Check sheet for the modelled part. Datum: model origin and axes. Units: mm. Face numbers are marked on the shaded views. A direction names the side the tool comes from. Give positions to 0.01 mm unless a question says otherwise; leave off trailing zeros. Order: outer loops, then holes, each group sorted by start corner. A loop starts at its lowest first (then second) coordinate and runs counter-clockwise, first axis right, second up. Notation, with made-up numbers: (-31, 79) -> (-3, 79) arc R14 ccw to (-3, 88) -> close; hole circle Ø4 at (-0.75, 50). An arc over 180 degrees is marked (long way). One line per question, with ' | ' between items. Start each with the question number.
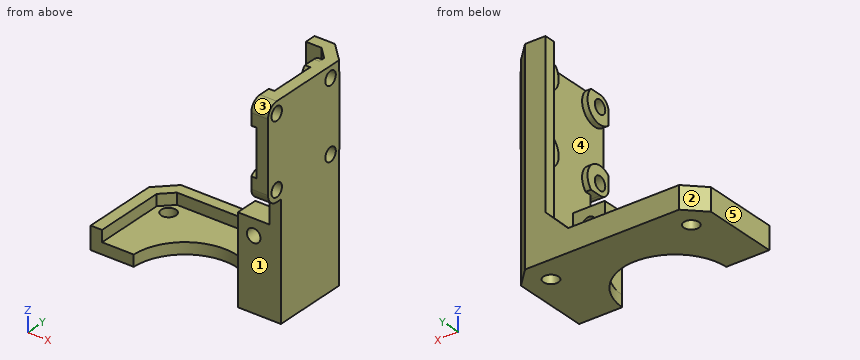
from build123d import *

# Parameters (mm, degrees)
BOSS_EXTRUDE1_DEPTH     = 2.5
SKETCH2_R               = 11.5
CUT_EXTRUDE1_DEPTH      = 3
SKETCH3_R               = 1.65
CUT_EXTRUDE2_DEPTH      = 3
EXTRUDE_THIN1_DEPTH     = 43.3
BOSS_EXTRUDE2_DEPTH     = 2.5
CUT_EXTRUDE3_DEPTH      = 57.003950753
CUT_EXTRUDE3_DEPTH_BACK = 57.003950753
SKETCH7_W               = 33.5
SKETCH7_H               = 40.8
CHAMFER1_SIZE           = 5
BOSS_EXTRUDE3_DEPTH     = 1.2
SKETCH10_R              = 1.5
CUT_EXTRUDE4_DEPTH      = 10
SKETCH12_W              = 9.502717712
SKETCH12_H              = 19.3
BOSS_EXTRUDE4_DEPTH     = 5
SKETCH13_R              = 1.5
CUT_EXTRUDE5_DEPTH      = 53.789227121


with BuildPart() as part:
    # Sketch1 → Boss-Extrude1 (new body)
    with BuildSketch(Plane.XY):
        Polygon((-21, 0.25), (21, 0.25), (21, 17), (17, 21), (-17, 21), (-21, 17), align=None)
    extrude(amount=BOSS_EXTRUDE1_DEPTH)

    # Sketch2 → Cut-Extrude1 (cut)
    with BuildSketch(Plane.XY.offset(2.5)):
        Circle(SKETCH2_R)
    extrude(amount=-CUT_EXTRUDE1_DEPTH, mode=Mode.SUBTRACT)

    # Sketch3 → Cut-Extrude2 (cut)
    with BuildSketch(Plane(origin=(0, 0, 0), x_dir=(-1, 0, 0), z_dir=(0, 0, -1))):
        with Locations((15.5, 15.5)):
            Circle(SKETCH3_R)
        with Locations((-15.5, 15.5)):
            Circle(SKETCH3_R)
    extrude(amount=-CUT_EXTRUDE2_DEPTH, mode=Mode.SUBTRACT)

    # Sketch4 → Extrude-Thin1 (add)
    with BuildSketch(Plane.XY.offset(2.5)):
        Polygon((21, 0.25), (21, 17), (17, 21), (-17, 21), (-21, 17), (-21, 0.25), (-18.5, 0.25), (-18.5, 15.964466094), (-15.964466094, 18.5), (15.964466094, 18.5), (18.5, 15.964466094), (18.5, 0.25), align=None)
    extrude(amount=EXTRUDE_THIN1_DEPTH)

    # Sketch6 → Boss-Extrude2 (add)
    with BuildSketch(Plane(origin=(21, 0, 0), x_dir=(0, 0, -1), z_dir=(1, 0, 0))):
        with BuildLine():
            Line((-45.8, 14.55), (-45.8, -0.95))
            ThreePointArc((-45.8, -0.95), (-45.067766953, -2.717766953), (-43.3, -3.45))
            Line((-43.3, -3.45), (-27.8, -3.45))
            ThreePointArc((-27.8, -3.45), (-26.032233047, -2.717766953), (-25.3, -0.95))
            Line((-25.3, -0.95), (-25.3, 14.55))
            ThreePointArc((-25.3, 14.55), (-26.032233047, 16.317766953), (-27.8, 17.05))
            Line((-27.8, 17.05), (-43.3, 17.05))
            ThreePointArc((-43.3, 17.05), (-45.067766953, 16.317766953), (-45.8, 14.55))
        make_face()
    extrude(amount=-BOSS_EXTRUDE2_DEPTH)

    # Sketch7 → Cut-Extrude3 (cut, two sides: drawn at the far end of the back side and taken through both)
    with BuildSketch(Plane(origin=(0, 21, 0), x_dir=(1, 0, 0), z_dir=(0, 1, 0)).offset(-CUT_EXTRUDE3_DEPTH_BACK)):
        with Locations((-4.25, -25.4)):
            Rectangle(SKETCH7_W, SKETCH7_H)
    extrude(amount=CUT_EXTRUDE3_DEPTH + CUT_EXTRUDE3_DEPTH_BACK, mode=Mode.SUBTRACT)

    # Chamfer1
    chamfer1_edges = [part.edges().sort_by_distance(p)[0] for p in [
        (12.5, 19.75, 5),
    ]]
    chamfer(chamfer1_edges, length=CHAMFER1_SIZE)

    # Sketch8 → Boss-Extrude3 (add)
    with BuildSketch(Plane.ZY.offset(-18.5)):
        with BuildLine():
            Line((27.8, -3.45), (30.390366769, -3.45))
            ThreePointArc((30.390366769, -3.45), (30.345584412, 1.595584412), (25.3, 1.640366769))
            Line((25.3, 1.640366769), (25.3, -0.95))
            ThreePointArc((25.3, -0.95), (26.032233047, -2.717766953), (27.8, -3.45))
        make_face()
        with BuildLine():
            Line((45.8, -0.95), (45.8, 1.640366769))
            ThreePointArc((45.8, 1.640366769), (40.754415588, 1.595584412), (40.709633231, -3.45))
            Line((40.709633231, -3.45), (43.3, -3.45))
            ThreePointArc((43.3, -3.45), (45.067766953, -2.717766953), (45.8, -0.95))
        make_face()
        with BuildLine():
            Line((43.3, 17.05), (40.709633231, 17.05))
            ThreePointArc((40.709633231, 17.05), (40.754415588, 12.004415588), (45.8, 11.959633231))
            Line((45.8, 11.959633231), (45.8, 14.55))
            ThreePointArc((45.8, 14.55), (45.067766953, 16.317766953), (43.3, 17.05))
        make_face()
        with BuildLine():
            Line((25.3, 14.55), (25.3, 11.959633231))
            ThreePointArc((25.3, 11.959633231), (30.345584412, 12.004415588), (30.390366769, 17.05))
            Line((30.390366769, 17.05), (27.8, 17.05))
            ThreePointArc((27.8, 17.05), (26.032233047, 16.317766953), (25.3, 14.55))
        make_face()
    extrude(amount=BOSS_EXTRUDE3_DEPTH)

    # Sketch10 → Cut-Extrude4 (cut)
    with BuildSketch(Plane.ZY.offset(-17.3)):
        with Locations((43.3, 14.55)):
            Circle(SKETCH10_R)
        with Locations((27.8, 14.55)):
            Circle(SKETCH10_R)
        with Locations((27.8, -0.95)):
            Circle(SKETCH10_R)
        with Locations((43.3, -0.95)):
            Circle(SKETCH10_R)
    extrude(amount=-CUT_EXTRUDE4_DEPTH, mode=Mode.SUBTRACT)

    # Sketch12 → Boss-Extrude4 (add)
    with BuildSketch(Plane.XZ.offset(-0.25)):
        with Locations((16.248641144, 9.65)):
            Rectangle(SKETCH12_W, SKETCH12_H)
    extrude(amount=-BOSS_EXTRUDE4_DEPTH)

    # Sketch13 → Cut-Extrude5 (cut, through all)
    with BuildSketch(Plane(origin=(0, 5.25, 0), x_dir=(1, 0, 0), z_dir=(0, 1, 0))):
        with Locations(Location((14.998641144, -15.8, 0), (0, 0, 270))):
            Circle(SKETCH13_R)
    extrude(amount=-CUT_EXTRUDE5_DEPTH, mode=Mode.SUBTRACT)


solid = part.part
1. Tool access check on the marked faces 1 and 2. Record the directions out of +Z, -Z, +X, -X, +Y, -Y that give a thin tool (end or side, any length) a straight path to the whole face; none if there is none.
2. Cross-section at C-C on x = 0. Record the boundary of the cut face in (y, z).
3. Cross-section at B-B on y = 4.5. Record the boundary of the cut face in (x, z), and give its area (3 significant figures).
4. Go/stop test with flat-tipped pins: pin 1 (6 mm diameter, centred on x = -2, y = 12.5, fed in from +Z); pin 2 (3 mm diameter, centred on y = 2.5, z = 30, fed in from -X); pin 3 (5 mm diameter, centred on x = 15, y = 7.5, fed in from +Z); pin 4 (8 mm diameter, centred on x = -15, y = 8, fed in from -Z). Record where each tip stops, or that it passes through.
5. Cross-section at D-D on z = 32. Record the boundary of the cut face in (x, y).
6. Cross-section at A-A on z = 15.8. Record the boundary of the cut face in (x, y), and give its area (3 significant figures).
7. Mould release check, pull along Z, two halves, no side actions. Record for the marked faces 3, 4 and 5: +Z half, -Z half, draft (parallel to the pull), parting line (faces both ways), or undercut.
8. Scan lines: probe 1 along X at (y, z) = (1, 3); probe 2 along X at (y, z) = (11.25, 4.5); probe 3 along Y at (x, z) = (15.5, 1.15). Record each from-to range of solid material in increasing order.
Response values:
1) face 1: -Z, +X, -X, -Y | face 2: +Z, -Z, -X, +Y
2) outline: (11.5, 0) -> (21, 0) -> (21, 5) -> (18.5, 5) -> (18.5, 2.5) -> (11.5, 2.5) -> close
3) outline: (-21, 0) -> (-10.58, 0) -> (-10.58, 2.5) -> (-18.5, 2.5) -> (-18.5, 5) -> (-21, 5) -> close; (10.58, 0) -> (21, 0) -> (21, 45.8) -> (18.5, 45.8) -> (18.5, 19.3) -> (11.5, 19.3) -> (11.5, 2.5) -> (10.58, 2.5) -> close; hole circle Ø3 at (15, 15.8) | area: 277 mm²
4) pin 1: stops at z = 2.5 | pin 2: stops at x = 17.3 | pin 3: stops at z = 19.3 | pin 4: stops at z = 0
5) outline: (12.5, 18.5) -> (15.96, 18.5) -> (18.5, 15.96) -> (18.5, -3.45) -> (21, -3.45) -> (21, 17.05) -> (20.95, 17.05) -> (17, 21) -> (12.5, 21) -> close
6) outline: (11.5, 0.25) -> (13.5, 0.25) -> (13.5, 5.25) -> (11.5, 5.25) -> close; (12.5, 18.5) -> (15.96, 18.5) -> (18.5, 15.96) -> (18.5, 5.25) -> (16.5, 5.25) -> (16.5, 0.25) -> (21, 0.25) -> (21, 17) -> (17, 21) -> (12.5, 21) -> close | area: 82.1 mm²
7) face 3: +Z half | face 4: undercut | face 5: draft
8) probe 1: x = -21 to -18.5, 11.5 to 21 | probe 2: x = -21 to -18.5, 18.5 to 21 | probe 3: y = 0.25 to 13.85, 17.15 to 21
